The listing builds one solid part. Answer for the finished solid, in the listing's coordinates (mm). A direction names the side the tool comes from. Give positions to 0.01 mm unless a question says otherwise; leave off trailing zeros. Write each loop counter-clockwise with the first axis right and the second up, starting at its lowest first coordinate (ties: lowest second). Pieces come first, ordered by that corner, then holes. Notation, with made-up numbers: (45.25, -35) - (57.25, -35) arc R24 cw to (57.25, -9) - close; hole circle Ø10 at (14, 51). An arc over 180 degrees is marked (long way). Use a Markdown table: item, result. Add a question column.
from build123d import *

# Parameters (mm, degrees)
F1_DEPTH  = 4.91
F2_R      = 0.7
F3_DEPTH  = 0.85
F6_DEPTH  = 0.6
F7_R      = 0.9
F8_DEPTH  = 0.6
F11_R     = 2
F12_DEPTH = 4
F15_W     = 5.8206040412
F15_H     = 6.0758944601
F16_DEPTH = 1.21


with BuildPart() as f1:
    # F0 (on Top) → F1 (new body)
    with BuildSketch(Plane.XY):
        with BuildLine():
            Line((-9.35, 9.3296706912), (-9.35, -8.25))
            Line((-9.35, -8.25), (9.65, -8.25))
            Line((9.65, -8.25), (9.65, 7.8709153458))
            Line((9.65, 7.8709153458), (10.25, 7.8709153458))
            ThreePointArc((10.25, 7.8709153458), (9.5849645406, 9.7831678774), (7.75, 10.6386718467))
            Line((7.75, 10.6386718467), (6.75, 9.85))
            Line((6.75, 9.85), (-6.6136931828, 9.85))
            ThreePointArc((-6.6136931828, 9.85), (-7.8763800086, 9.0352078731), (-9.35, 9.3296706912))
        make_face()
    extrude(amount=-F1_DEPTH)

    # F2 (on face) → F3 (join)
    with BuildSketch(Plane.XY):
        with Locations((-7.5, -6.8)):
            Circle(F2_R)
        with Locations((7.5, -6.8)):
            Circle(F2_R)
        with Locations((-7.5, 6.8)):
            Circle(F2_R)
        with Locations((7.5, 6.8)):
            Circle(F2_R)
    extrude(amount=F3_DEPTH)

    # F5 (on offset) → F6 (join)
    with BuildSketch(Plane.XY.offset(-3.1)):
        with BuildLine():
            Line((-10.25, 10.1498657733), (-9.0825001077, 8.6487947561))
            Line((-9.0825001077, 8.6487947561), (-6.25, 8.6487947561))
            Line((-6.25, 8.6487947561), (-6.25, 11))
            ThreePointArc((-6.25, 11), (-8.25, 13), (-10.25, 11))
            Line((-10.25, 11), (-10.25, 10.1498657733))
        make_face()
        with BuildLine():
            Line((7.75, 11), (7.75, 8.4319217131))
            Line((7.75, 8.4319217131), (9.9920006469, 8.4319217131))
            Line((9.9920006469, 8.4319217131), (11.75, 10.1568773389))
            Line((11.75, 10.1568773389), (11.75, 11))
            ThreePointArc((11.75, 11), (9.75, 13), (7.75, 11))
        make_face()
    extrude(amount=-F6_DEPTH)

    # F7 (on face) → F8 (cut, through all)
    with BuildSketch(Plane.XY.offset(-3.1)):
        with Locations((-8.25, 11)):
            Circle(F7_R)
        with Locations((9.75, 11)):
            Circle(F7_R)
    extrude(amount=-F8_DEPTH, mode=Mode.SUBTRACT)

    # F9 (on Front) → F10 (revolve)
    with BuildSketch(Plane.XZ):
        with BuildLine():
            Line((3.1952585559, 2.2070568521), (0, 2.2070568521))
            Line((0, 2.2070568521), (0, 0))
            Line((0, 0), (6.177762989, 0))
            ThreePointArc((6.177762989, 0), (5.0504157353, 1.5952910936), (3.1952585559, 2.2070568521))
        make_face()
    revolve(axis=Axis((0, 0, 1.103528426), (0, 0, -1)))

    # F11 (on face) → F12 (cut)
    with BuildSketch(Plane.XY.offset(2.2070568521)):
        Circle(F11_R)
    extrude(amount=-F12_DEPTH, mode=Mode.SUBTRACT)

    # F13 (on Front) → F14 (revolve)
    with BuildSketch(Plane.XZ):
        with BuildLine():
            Line((0, 6.9), (0, -2))
            Line((0, -2), (2, -2))
            Line((2, -2), (2, 5))
            Line((2, 5), (6, 5))
            Line((6, 5), (6, 5.8))
            ThreePointArc((6, 5.8), (4.3343936328, 6.6185251952), (2.5, 6.9))
            Line((2.5, 6.9), (0, 6.9))
        make_face()
    revolve(axis=Axis((0, 0, 2.45), (0, 0, 1)))

    # F15 (on face) → F16 (cut, through all)
    with BuildSketch(Plane(origin=(0, 0, -4.91), x_dir=(1, 0, 0), z_dir=(0, 0, -1))):
        with Locations((7.839627564, -7.8769084066)):
            Rectangle(F15_W, F15_H)
    extrude(amount=-F16_DEPTH, mode=Mode.SUBTRACT)


solid = f1.part
1. The part is cut by section A-A (y = 6.8). Give the vertices of the cut face in (x, z).
2. Which of the six approach directions +Z, -Z, +X, -X, +Y, -Y give full straight-line access (tool end or side, diameter ignored) to faces 5 (the flat face through (-3, 0, 5)), 6 (the flat face through (7, -7, 0.85)), 7 (the flat face through (5, 6, 0)), 8 (the flat face through (8, 9, -3.7)), 9 (the flat face through (11, 11, -3.1))?
3. Consider L1, parallel to Y at x = -8.25, z = -3.5; L2, parallel to Z at x = 8, y = -7; L3, parallel to X at y = -4.75, z = -1.25. Determine where each line is inside the solid, lowest interval first. Write a range as [from, to].
4. For a pull along Y with two mould halves and no side action, classify faces 1 (the cylindrical face through (-8.2, 6.8, 0.4)), 2 (the cylindrical face through (-8.37, 11.89, -3.4)), 3 (the flat face through (0, 1, -4.91)), 4 (the cylindrical face through (-5.994, 0.264, 5.406)) as released by +Y, released by -Y, zero draft, split by the parting line, or undercut.
5. Given P1, Ø1.5, axis at x = 2, z = -2.5, coming from the +Y side; P2, Ø5.5, axis at x = 10, y = 8, coming from the -Z side; P3, Ø4, axis at x = 1.5, z = 3.5, coming from the -Y side; P4, Ø1.4, axis at x = -8.25, y = 11, coming from the -Z side, each flat-ended and moving along its own axis, determine where each tip first touches the part or whether it passes through.
6. The part is cut by section C-C (z = 1.5). Give the vertices of the cut face in (x, y).
7. The part is cut by section B-B (z = -1). Give the vertices of the cut face in (x, y), and give its area (3 significant figures).
Check values:
| question | item | result |
|---|---|---|
| 1 | outline | (-9.35, -4.91) - (4.93, -4.91) - (4.93, -3.7) - (9.65, -3.7) - (9.65, 0) - (8.2, 0) - (8.2, 0.85) - (6.8, 0.85) - (6.8, 0) - (-6.8, 0) - (-6.8, 0.85) - (-8.2, 0.85) - (-8.2, 0) - (-9.35, 0) - close |
| 2 | face 5 | none |
| 2 | face 6 | +Z, +X, -X, +Y, -Y |
| 2 | face 7 | +Z |
| 2 | face 8 | -Z, +X, +Y |
| 2 | face 9 | +Z, +X, +Y |
| 3 | L1 | y = [-8.25, 10.1], [11.9, 13] |
| 3 | L2 | z = [-4.91, 0.85] |
| 3 | L3 | x = [-9.35, 9.65] |
| 4 | face 1 | undercut |
| 4 | face 2 | undercut |
| 4 | face 3 | zero draft |
| 4 | face 4 | split by the parting line |
| 5 | P1 | stops at y = 9.85 |
| 5 | P2 | stops at z = -3.7 |
| 5 | P3 | stops at y = -6 |
| 5 | P4 | passes through |
| 6 | outline | circle Ø10.35 at (0, 0) |
| 7 | outline | (-9.35, -8.25) - (9.65, -8.25) - (9.65, 7.87) - (10.25, 7.87) arc R2.6 ccw to (7.75, 10.64) - (6.75, 9.85) - (-6.61, 9.85) arc R2 cw to (-9.35, 9.33) - close |
| 7 | area | 344 mm2 |
